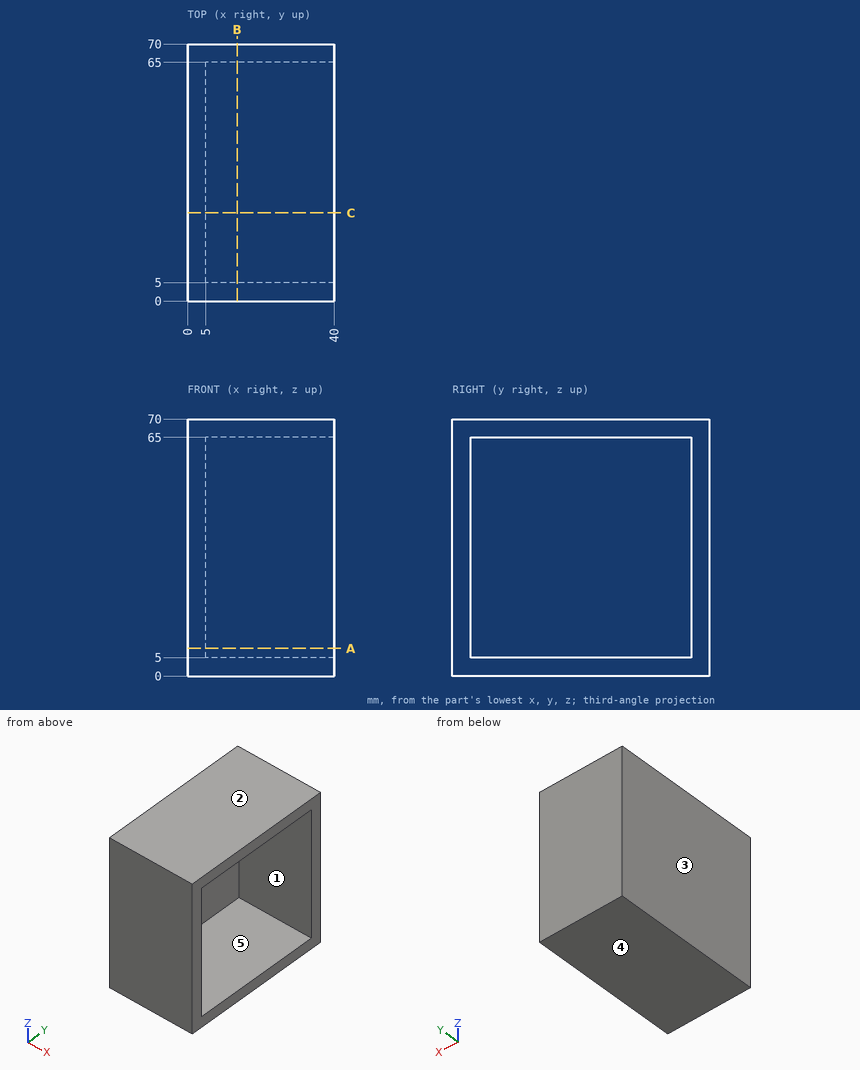
The figure shows three views and two pictorial views of one solid part (mm, origin at its lowest corner). Answer the questions. A direction names the side the tool comes from. Round coordinates to 2 decimals unless told otherwise and drop trailing zeros. Write each loop counter-clockwise with the first axis right and the second up, starting at its lowest first coordinate (ties: lowest second). Pieces come first, ordered by that corner, then holes. Notation, with made-up numbers: (43, 58) - (86, 58) arc R6 ccw to (86, 66) - close; hole circle Ø10 at (67, 22). An arc over 180 degrees is marked (long way). Use one line per item in the form item = value. Start each with the question number.
Item 1: A cutting plane is placed at A-A (z = 7.5). Write down the section's boundary in (x, y).
Item 2: A tool of negligible diameter and unlimited length cuts with its end or side. For the marked faces 4 and 5, from which of +Z, -Z, +X, -X, +Y, -Y can it reach the whole face along a straight path? Write none if from no direction.
Item 3: Determine the mould class of the marked faces 1, 2 and 3 for opening direction Z: +Z half, -Z half, draft (parallel to the pull), parting line (faces both ways), or undercut.
Item 4: Find the intervals of material crossed by line 1 (Z direction, x = 17.5, y = 61.5); line 2 (X direction, y = 31, z = 41), in increasing order. Write a range as [from, to].
Item 5: A cutting plane is placed at B-B (x = 13.5). Write down the section's boundary in (y, z), plus the area to 3 significant figures.
Item 6: A flat-ended cylindrical pin translates along its axis: pin 1 Ø1 at (y, z) = (47, 31.5) entering from +X. Find the tip coordinate at first contact, or state that the pin passes through.
The answers:
q1.outline = (0, 0) - (40, 0) - (40, 5) - (5, 5) - (5, 65) - (40, 65) - (40, 70) - (0, 70) - close
q2.face_4 = -Z, +X, -X, +Y, -Y
q2.face_5 = +X
q3.face_1 = undercut
q3.face_2 = +Z half
q3.face_3 = draft
q4.line_1 = [0, 5], [65, 70]
q4.line_2 = [0, 5]
q5.outline = (0, 0) - (70, 0) - (70, 70) - (0, 70) - close; hole (5, 5) - (65, 5) - (65, 65) - (5, 65) - close
q5.area = 1,300 mm^2
q6.pin_1 = 5
